```python
from build123d import *

# Parameters (mm, degrees)
SKETCH2_R           = 1.625
SKETCH2_R_2         = 11.5
SKETCH2_R_3         = 2
SKETCH2_R_4         = 1.5
SKETCH2_W           = 30
SKETCH2_H           = 4.5
SKETCH2_W_2         = 4.5
SKETCH2_H_2         = 30
BOSS_EXTRUDE1_DEPTH = 5


with BuildPart() as part:
    # Sketch2 → Boss-Extrude1 (new body)
    with BuildSketch(Plane(origin=(0, 0, 0), x_dir=(1, 0, 0), z_dir=(0, 1, 0))):
        with BuildLine():
            Line((-120, 42.726979343), (-120, 102.67073807))
            Line((-120, 102.67073807), (-150.055809303, 102.67073807))
            Line((-150.055809303, 102.67073807), (-150.055809303, -106.82926193))
            Line((-150.055809303, -106.82926193), (-136.055809303, -106.82926193))
            Line((-136.055809303, -106.82926193), (-136.055809303, -177.32926193))
            Line((-136.055809303, -177.32926193), (136.055809303, -177.32926193))
            Line((136.055809303, -177.32926193), (136.055809303, -106.82926193))
            Line((136.055809303, -106.82926193), (150.055809303, -106.82926193))
            Line((150.055809303, -106.82926193), (150.055809303, 102.923994861))
            Line((150.055809303, 102.923994861), (120, 102.923994861))
            Line((120, 102.923994861), (120, 87.604878279))
            Line((120, 87.604878279), (120, 42.726979343))
            ThreePointArc((120, 42.726979343), (117.955549577, 27.197836637), (111.961524227, 12.726979343))
            Line((111.961524227, 12.726979343), (51.961524227, -91.196069111))
            ThreePointArc((51.961524227, -91.196069111), (0, -121.196069111), (-51.961524227, -91.196069111))
            Line((-51.961524227, -91.196069111), (-111.961524227, 12.726979343))
            ThreePointArc((-111.961524227, 12.726979343), (-117.955549577, 27.197836637), (-120, 42.726979343))
        make_face()
        with Locations(Location((-143.555809303, 2.104507355, 0), (0, 0, 270))):
            Circle(SKETCH2_R, mode=Mode.SUBTRACT)
        with Locations(Location((-115.5, 2.104507355, 0), (0, 0, 270))):
            Circle(SKETCH2_R, mode=Mode.SUBTRACT)
        with Locations(Location((115.5, 2.104507355, 0), (0, 0, 270))):
            Circle(SKETCH2_R, mode=Mode.SUBTRACT)
        with Locations(Location((143.555809303, 2.104507355, 0), (0, 0, 270))):
            Circle(SKETCH2_R, mode=Mode.SUBTRACT)
        with Locations(Location((129.555809303, 2.201175016, 0), (0, 0, 270))):
            Circle(SKETCH2_R_2, mode=Mode.SUBTRACT)
        with Locations(Location((-129.555809303, 2.201175016, 0), (0, 0, 270))):
            Circle(SKETCH2_R_2, mode=Mode.SUBTRACT)
        with Locations(Location((-125, -135.82926193, 0), (0, 0, 270))):
            Circle(SKETCH2_R_3, mode=Mode.SUBTRACT)
        with Locations(Location((-125, -148.32926193, 0), (0, 0, 270))):
            Circle(SKETCH2_R_3, mode=Mode.SUBTRACT)
        with Locations(Location((-80, -135.82926193, 0), (0, 0, 270))):
            Circle(SKETCH2_R_3, mode=Mode.SUBTRACT)
        with Locations(Location((-80, -148.32926193, 0), (0, 0, 270))):
            Circle(SKETCH2_R_3, mode=Mode.SUBTRACT)
        with Locations(Location((80, -135.82926193, 0), (0, 0, 270))):
            Circle(SKETCH2_R_3, mode=Mode.SUBTRACT)
        with Locations(Location((80, -148.32926193, 0), (0, 0, 270))):
            Circle(SKETCH2_R_3, mode=Mode.SUBTRACT)
        with Locations(Location((125, -148.32926193, 0), (0, 0, 270))):
            Circle(SKETCH2_R_3, mode=Mode.SUBTRACT)
        with Locations(Location((125, -135.82926193, 0), (0, 0, 270))):
            Circle(SKETCH2_R_3, mode=Mode.SUBTRACT)
        with Locations(Location((-135.027904651, 86.57073807, 0), (0, 0, 270))):
            Circle(SKETCH2_R_4, mode=Mode.SUBTRACT)
        with Locations(Location((-135.027904651, 76.57073807, 0), (0, 0, 270))):
            Circle(SKETCH2_R_4, mode=Mode.SUBTRACT)
        with Locations(Location((135.027904651, 76.57073807, 0), (0, 0, 270))):
            Circle(SKETCH2_R_4, mode=Mode.SUBTRACT)
        with Locations(Location((135.027904651, 86.57073807, 0), (0, 0, 270))):
            Circle(SKETCH2_R_4, mode=Mode.SUBTRACT)
        with Locations(Location((-135.027904651, 57.67073807, 0), (0, 0, 270))):
            Circle(SKETCH2_R_4, mode=Mode.SUBTRACT)
        with Locations(Location((135.027904651, 57.67073807, 0), (0, 0, 270))):
            Circle(SKETCH2_R_4, mode=Mode.SUBTRACT)
        with Locations(Location((66.055809303, -167.32926193, 0), (0, 0, 270))):
            Circle(SKETCH2_R_4, mode=Mode.SUBTRACT)
        with Locations(Location((-66.055809303, -167.32926193, 0), (0, 0, 270))):
            Circle(SKETCH2_R_4, mode=Mode.SUBTRACT)
        with Locations((-20, -170.07926193)):
            Rectangle(SKETCH2_W, SKETCH2_H, mode=Mode.SUBTRACT)
        with Locations((20, -170.07926193)):
            Rectangle(SKETCH2_W, SKETCH2_H, mode=Mode.SUBTRACT)
        with Locations((142.805809303, -81.82926193)):
            Rectangle(SKETCH2_W_2, SKETCH2_H_2, mode=Mode.SUBTRACT)
        with Locations((142.805809303, -41.82926193)):
            Rectangle(SKETCH2_W_2, SKETCH2_H_2, mode=Mode.SUBTRACT)
        with Locations((-142.805809303, -81.82926193)):
            Rectangle(SKETCH2_W_2, SKETCH2_H_2, mode=Mode.SUBTRACT)
        with Locations((-142.805809303, -41.82926193)):
            Rectangle(SKETCH2_W_2, SKETCH2_H_2, mode=Mode.SUBTRACT)
    extrude(amount=BOSS_EXTRUDE1_DEPTH)


solid = part.part
```
Can you work these out from the model? Positions are in its coordinate system, mm. A direction names the side the tool comes from. Coordinates: 2 decimals unless noted, no trailing zeros. Loops run counter-clockwise (first coordinate to the right, second up) from the corner with the lowest first, then second, coordinate; pieces in that order, holes last.
1) Thinking about a two-plate mould opening in X: for faces 3 (the cylindrical face through (0.88, 2.46, 121.19)), 4 (the cylindrical face through (-140.782, 2.465, -4.694)), 5 (the flat face through (-2, 0, 129)), which applies, pulls with the +X half, pulls with the -X half, needs draft (parallel to the pull), parting line crosses it, or undercut?
2) For pin 1 (2.5 mm diameter, centred on x = -134, y = 3.5, fed in from -Z); pin 2 (2 mm diameter, centred on x = 143.5, y = 1.5, fed in from +Z); pin 3 (1.5 mm diameter, centred on y = 1, z = 126.5, fed in from +X), each with a flat end and sliding along its axis, tell me the tip position at first contact or that it passes through.
3) Imagine slicing it at C-C on y = 1.25. State how many separate pieces and enclosed holes the cut face has, plus the area to 3 significant figures.
4) I need wall thicknesses on probe 1 along X at (y, z) = (3.5, -85); probe 2 along Z at (x, y) = (-66, 2.7); probe 3 along X at (y, z) = (0.8, 3). Which ranges of each line are inside material? Lowest first, please.
5) Imagine slicing it at B-B on x = -45.5. List the corners of the cut face in (y, z) for me.
6) Which directions (+Z, -Z, +X, -X, +Y, -Y) give clear straight access to the entire face, cutting with the end or side of a thin tool? Please do faces 1 (the flat face through (-2, 5, 129)), 2 (the cylindrical face through (118.01, 2.46, -27.41)).
7) Imagine slicing it at A-A on z = 79. List the corners of the cut face in (x, y) for me.
Completed:
1. face 3: undercut
1. face 4: undercut
1. face 5: needs draft
2. pin 1: stops at z = -102.67
2. pin 2: stops at z = 106.83
2. pin 3: stops at x = 136.06
3. separate pieces: 1
3. enclosed holes: 28
3. area: 39,600 mm2
4. probe 1: x = -150.06 to -120, 120 to 150.06
4. probe 2: z = 66.88 to 165.83, 168.83 to 177.33
4. probe 3: x = -150.06 to -139.81, -119.3 to -102.88, 102.88 to 119.3, 139.81 to 150.06
5. outline: (0, 100.31) - (5, 100.31) - (5, 177.33) - (0, 177.33) - close
6. face 1: +Z, -Z, +X, -X, +Y
6. face 2: -Z, +Y, -Y
7. outline: (-150.06, 0) - (-145.06, 0) - (-145.06, 5) - (-150.06, 5) - close; (-140.56, 0) - (-59, 0) - (-59, 5) - (-140.56, 5) - close; (59, 0) - (140.56, 0) - (140.56, 5) - (59, 5) - close; (145.06, 0) - (150.06, 0) - (150.06, 5) - (145.06, 5) - close
